Input: part model. Units: mm. Frame: model coordinates. A direction names the side the tool comes from. Coordinates: 2 decimals unless noted, no trailing zeros. Loops run counter-clockwise (first coordinate to the right, second up) from the corner with the lowest first, then second, coordinate; pieces in that order, holes last.
Autodesk Inventor part; units mm, degrees
ref_plane "YZ Plane" through (0, 0, 0) normal (1, 0, 0) x (0, 1, 0)
ref_plane "XZ Plane" through (0, 0, 0) normal (0, 1, 0) x (-1, 0, 0)
ref_plane "XY Plane" through (0, 0, 0) normal (0, 0, 1) x (1, 0, 0)
sketch "Skizze1" plane through (0, 0, 0) normal (1, 0, 0) x (0, 1, 0)
  line L0 (5, -20) -> (5, -25)
  line L1 (5, -20) -> (0, -20)
  line L2 (0, -20) -> (0, -55)
  line L3 (0, -55) -> (5, -55)
  line L4 (5, -55) -> (5, -20)
  line L5 (0, -42) -> (0, -47)
  line L6 (0, -37.5) -> (0, -42)
  line L7 (-8, 0) -> (13, 0)
  line L8 (0, -66) -> (0, 11)
  line L9 (5, -20) -> (0, -20)
  line L10 (0, -20) -> (0, 0)
  line L11 (0, 0) -> (5, 0)
  line L12 (5, 0) -> (5, -20)
  line L13 (-5, 0) -> (0, 0)
  line L14 (0, 0) -> (0, -47)
  line L15 (0, -47) -> (-5, -47)
  line L16 (-5, -47) -> (-5, 0)
  point P0 (10, -25)
  point P1 (10, -20)
  point P2 (0, -44.5)
  point P3 (2.5, -55)
  point P4 (-2.5, -47)
  dimension "d1" = 5
  dimension "d10" = 0
  dimension "d26" = 5
  dimension "d27" = 47
revolve "Umdrehung1" add sketch "Skizze1" angle 360 about axis through (0, -10, 0) along (0, 1, 0)
sketch "Skizze2" plane through (0, 5, 0) normal (0, 1, 0) x (1, 0, 0)
  line L0 (-77, 0) -> (77, 0)
  line L1 (0, 77) -> (0, -77)
  circle A0 centre (0, 0) radius 51
  circle A1 centre (0, 0) radius 55
  point P0 (0, -51)
  point P1 (44.1673, -25.5)
  point P2 (44.1673, 25.5)
  point P3 (0, 51)
  point P4 (-44.1673, 25.5)
  point P5 (-44.1673, -25.5)
  dimension "d14" = 4
  dimension "d17" = 360
hole "Bohrung1" at (0, 5, 51) at (44.1673, 5, 25.5) at (44.1673, 5, -25.5) at (0, 5, -51) at (-44.1673, 5, -25.5) at (-44.1673, 5, 25.5) direction (0, -1, 0) diameter 4.5 depth 11.8 tip angle 118
properties part number "Deckel Stempel 2"
Item 1: Section query B-B (y = 1.75). Output: boundary loops of the cut face in (x, z).
Result:
outline: circle Ø110 at (0, 0); hole circle Ø4.5 at (-44.17, -25.5); hole circle Ø4.5 at (-44.17, 25.5); hole circle Ø4.5 at (0, -51); hole circle Ø4.5 at (0, 51); hole circle Ø4.5 at (44.17, -25.5); hole circle Ø4.5 at (44.17, 25.5)
Item 2: Section query C-C (z = -51). Output: boundary loops of the cut face in (x, y), then the cut area to 3 significant figures.
Result:
outline: (-20.59, 0) - (-2.25, 0) - (-2.25, 5) - (-20.59, 5) - close; (2.25, 0) - (20.59, 0) - (20.59, 5) - (2.25, 5) - close
area: 183 mm2
Item 3: Line query: L1, parallel to X at y = 3.1, z = 25.5; L2, parallel to Z at x = 0, y = 3.85; L3, parallel to Y at x = -45, z = 20.5. Output: solid intervals per line, ascending.
Result:
L1: x = -48.73 to -46.42, -41.92 to 41.92, 46.42 to 48.73
L2: z = -55 to -53.25, -48.75 to 48.75, 53.25 to 55
L3: y = 0 to 5
Item 4: Reachability of faces 1 (the face through (-42.17, 2.46, 26.54)), 2 (the face through (40.5, 0, -24.2)) from +Z, -Z, +X, -X, +Y, -Y: full face, straight path, thin tool, end or side. Return the list, or none.
Result:
face 1: +Y, -Y
face 2: -Y
Item 5: Section query D-D (z = -12). Output: boundary loops of the cut face in (x, y).
Result:
outline: (-53.67, 0) - (-45.44, 0) - (-45.44, -5) - (45.44, -5) - (45.44, 0) - (53.67, 0) - (53.67, 5) - (-53.67, 5) - close
Item 6: Section query A-A (z = -26.5). Output: boundary loops of the cut face in (x, y).
Result:
outline: (-48.19, 0) - (-46.18, 0) - (-46.18, 5) - (-48.19, 5) - close; (-42.15, 0) - (-38.82, 0) - (-38.82, -5) - (38.82, -5) - (38.82, 0) - (42.15, 0) - (42.15, 5) - (-42.15, 5) - close; (46.18, 0) - (48.19, 0) - (48.19, 5) - (46.18, 5) - close
Item 7: Mould query, pull axis X, two halves, no side actions, for faces 3 (the face through (-0.099, 2.465, 48.752)), 4 (the face through (-1, -5, 1)), 5 (the face through (14.12, -2.54, -44.83)). Classes: +X half, -X half, draft (parallel to the pull), parting line (faces both ways), or undercut.
Result:
face 3: undercut
face 4: draft
face 5: parting line
Item 8: Contact query for flat-ended pins moving along their axis: P1, Ø4, axis at x = 30.5, y = -3, coming from the -Z side; P2, Ø6, axis at x = 0, z = 51, coming from the -Y side; P3, Ø4, axis at y = 3, z = 37.5, coming from the -X side; P4, Ø6, axis at x = 44.17, z = -25.5, coming from the +Y side. Output: stop coordinate, or through.
Result:
P1: stops at z = -37.37
P2: stops at y = 0
P3: stops at x = -42.01
P4: stops at y = 5
